from build123d import *

# Parameters (mm, degrees)
PAD_DEPTH           = 20
SKETCH001_R         = 2.6
POCKET_DEPTH        = 100
POCKET001_DEPTH     = 40
PAD001_DEPTH        = 70.3
SKETCH004_R         = 2.6
POCKET002_DEPTH     = 10
SKETCH005_R         = 2.6
POCKET003_DEPTH     = 10
SKETCH006_W         = 10
SKETCH006_H         = 1
POCKET004_DEPTH     = 25
SKETCH007_W         = 16.8
SKETCH007_H         = 35
PAD002_DEPTH        = 5.8
SKETCH008_W         = 12.8
SKETCH008_H         = 6
POCKET005_DEPTH     = 5.8
SKETCH009_W         = 16.8
SKETCH009_H         = 2
PAD003_DEPTH        = 15
SKETCH010_R         = 2
POCKET006_DEPTH     = 40
LINEARPATTERN_COUNT = 3
LINEARPATTERN_PITCH = 6
SKETCH011_R         = 1.6
POCKET007_DEPTH     = 12


with BuildPart() as part:
    # Sketch → Pad (new body)
    with BuildSketch(Plane.XZ):
        Polygon((17.1, 10.100008), (17.1, -4.899992), (25.3, -13.099992), (35.3, -13.099992), (35.3, -20.099992), (-35.3, -20.099992), (-35.3, -13.099992), (-25.3, -13.099992), (-17.1, -4.899992), (-17.1, 10.100008), (-17.1, 20.100008), (17.1, 20.100008), align=None)
        Polygon((-10.1, 10.100008), (-10.1, 4.900008), (-8.3, 3.099992), (-8.3, -3.100008), (-10.1, -4.899992), (-10.1, -10.099992), (-5.478931, -10.099992), (-5.478931, -11.099992), (5.478931, -11.099992), (5.478931, -10.099992), (10.1, -10.099992), (10.1, -4.899992), (8.3, -3.099992), (8.3, 3.100008), (10.1, 4.900008), (10.1, 10.100008), align=None, mode=Mode.SUBTRACT)
    extrude(amount=PAD_DEPTH)

    # Sketch001 (on Face22 of Pad) → Pocket (cut)
    with BuildSketch(Plane(origin=(8.3, 0, 0), x_dir=(0, 0, -1), z_dir=(-1, 0, 0))):
        with Locations((0, 10)):
            Circle(SKETCH001_R)
    extrude(amount=-POCKET_DEPTH, mode=Mode.SUBTRACT)

    # Sketch001 (on Face22 of Pad) → Pocket001 (cut)
    with BuildSketch(Plane(origin=(8.3, 0, 0), x_dir=(0, 0, -1), z_dir=(-1, 0, 0))):
        with Locations((0, 10)):
            Circle(SKETCH001_R)
    extrude(amount=POCKET001_DEPTH, mode=Mode.SUBTRACT)

    # Sketch003 → Pad001 (join)
    with BuildSketch(Plane(origin=(35.15, 0, 0), x_dir=(0, 0, 1), z_dir=(1, 0, 0))):
        Polygon((-20.000008, 14.8), (-20.000008, 5), (-21.800008, 6.8), (-21.800008, 13), align=None)
    extrude(amount=-PAD001_DEPTH)

    # Sketch004 (on Face3 of Pad001) → Pocket002 (cut)
    with BuildSketch(Plane(origin=(0, 0, -13.099992), x_dir=(-1, 0, 0), z_dir=(0, 0, 1))):
        with Locations((-30.3, 10)):
            Circle(SKETCH004_R)
    extrude(amount=-POCKET002_DEPTH, mode=Mode.SUBTRACT)

    # Sketch005 (on Face12 of Pocket002) → Pocket003 (cut)
    with BuildSketch(Plane(origin=(0, 0, -13.099992), x_dir=(-1, 0, 0), z_dir=(0, 0, 1))):
        with Locations((30.3, 10)):
            Circle(SKETCH005_R)
    extrude(amount=-POCKET003_DEPTH, mode=Mode.SUBTRACT)

    # Sketch006 (on Face4 of Pocket003) → Pocket004 (cut)
    with BuildSketch(Plane(origin=(0, 0, 0), x_dir=(1, 0, 0), z_dir=(0, 1, 0))):
        with Locations((0.1, -10.600008)):
            Rectangle(SKETCH006_W, SKETCH006_H)
    extrude(amount=-POCKET004_DEPTH, mode=Mode.SUBTRACT)

    # Sketch007 (on Face6 of Pocket004) → Pad002 (join)
    with BuildSketch(Plane(origin=(0, 0, 20.100008), x_dir=(-1, 0, 0), z_dir=(0, 0, 1))):
        with Locations((0, 2.5)):
            Rectangle(SKETCH007_W, SKETCH007_H)
    extrude(amount=PAD002_DEPTH)

    # Sketch008 (on Face46 of Pad002) → Pocket005 (cut)
    with BuildSketch(Plane(origin=(0, 0, 25.900008), x_dir=(-1, 0, 0), z_dir=(0, 0, 1))):
        with Locations((0, -12)):
            Rectangle(SKETCH008_W, SKETCH008_H)
    extrude(amount=-POCKET005_DEPTH, mode=Mode.SUBTRACT)

    # Sketch009 (on Face4 of Pocket005) → Pad003 (join)
    with BuildSketch(Plane(origin=(0, 0, 0), x_dir=(1, 0, 0), z_dir=(0, 1, 0))):
        with Locations((0, -19.100008)):
            Rectangle(SKETCH009_W, SKETCH009_H)
    extrude(amount=PAD003_DEPTH)

    # Sketch010 (on Face46 of Pad003) → Pocket006 (cut)
    with BuildSketch(Plane(origin=(0, 9, 0), x_dir=(1, 0, 0), z_dir=(0, 1, 0))):
        with Locations((-6.4, -23.000008)):
            Circle(SKETCH010_R)
    pocket006 = extrude(amount=-POCKET006_DEPTH, mode=Mode.SUBTRACT)

    # LinearPattern: Pocket006 ×3
    with Locations(*[(i * LINEARPATTERN_PITCH, 0, 0) for i in range(1, LINEARPATTERN_COUNT)]):
        add(pocket006, mode=Mode.SUBTRACT)

    # Sketch011 (on Face5 of LinearPattern) → Pocket007 (cut)
    with BuildSketch(Plane.XZ.offset(20)):
        with Locations((0, 16.970566)):
            Circle(SKETCH011_R)
    extrude(amount=-POCKET007_DEPTH, mode=Mode.SUBTRACT)


solid = part.part
Here's how the part is built. I have some questions about the finished solid (model axes, mm). A direction names the side the tool comes from. Coordinates: 2 decimals unless noted, no trailing zeros. Write each loop counter-clockwise with the first axis right and the second up, starting at its lowest first coordinate (ties: lowest second). Pieces come first, ordered by that corner, then holes. Notation, with made-up numbers: (-4.5, 15) - (19.5, 15) arc R14 ccw to (19.5, 34) - close; hole circle Ø5 at (23, 7). An arc over 180 degrees is marked (long way). Use one line per item in the form item = value.
1) Suppose I cut it at D-D, the plane x = 14. Write out the boundary of the cut face in (y, z), plus the area to 3 significant figures.
Solved:
outline = (-20, -20.1) - (-14.7, -20.1) - (-13, -21.8) - (-6.8, -21.8) - (-5.1, -20.1) - (0, -20.1) - (0, 20.1) - (-20, 20.1) - close; hole circle Ø5.2 at (-10, 0)
area = 796 mm2
2) On a 3-axis mill with a long thin cutter (end or side, diameter ignored), from which of +Z, -Z, +X, -X, +Y, -Y can I reach the whole of each face in a straight line? I mean faces 4 (the flat face through (-17.1, -10, 8)), 5 (the flat face through (0, 7, 18.1)), 6 (the flat face through (9.2, -9.9, 4)). Say none if no direction works.
Solved:
face_4 = +Z, -X, +Y, -Y
face_5 = -Z, +X, -X, +Y
face_6 = +Y, -Y
3) I'm going to push flat-ended pins straight in: P1, Ø5, axis at y = 0, z = 1.5, coming from the +X side; P2, Ø1.6, axis at y = -12.5, z = -8.5, coming from the -X side; P3, Ø6, axis at y = -12, z = 9.5, coming from the -X side. Where does each tip first touch, or does it pass through?
Solved:
P1 = 17.1
P2 = -21.5
P3 = -17.1
4) Suppose I cut it at A-A, the plane z = 6. Write out the boundary of the cut face in (x, y).
Solved:
outline = (-17.1, -20) - (-10.1, -20) - (-10.1, 0) - (-17.1, 0) - close; (10.1, -20) - (17.1, -20) - (17.1, 0) - (10.1, 0) - close
5) Thinking about a two-plate mould opening in Z: for faces 1 (the flat face through (8.4, -3, 22)), 2 (the cylindrical face through (-0.834, -5.297, 24.952)), 3 (the flat face through (21.1, -9.9, -8.9)), which applies, released by +Z, released by -Z, zero draft, split by the parting line, or undercut?
Solved:
face_1 = zero draft
face_2 = undercut
face_3 = released by +Z
6) Suppose I cut it at B-B, the plane x = -30.3. Write out the boundary of the cut face in (y, z), plus the area to 3 significant figures.
Solved:
outline = (-20, -20.1) - (-14.7, -20.1) - (-13, -21.8) - (-12.6, -21.8) - (-12.6, -13.1) - (-20, -13.1) - close; (-7.4, -21.8) - (-6.8, -21.8) - (-5.1, -20.1) - (0, -20.1) - (0, -13.1) - (-7.4, -13.1) - close
area = 108 mm2
7) I need wall thicknesses on line 1 (X direction, y = -10, z = -18); line 2 (Z direction, x = 5.6, y = -1); line 3 (Z direction, x = 12, y = -10). Which ranges of each line are inside material? Lowest first, please.
Solved:
line_1 = -35.3 to -32.9, -27.7 to 27.7, 32.9 to 35.3
line_2 = -20.1 to -10.1, 10.1 to 21, 25 to 25.9
line_3 = -21.8 to -2.6, 2.6 to 20.1
